from build123d import *

# Parameters (mm, degrees)
ESBO_O1_W                = 63
ESBO_O1_H                = 60
RESSALTO_EXTRUS_O1_DEPTH = 1
RESSALTO_EXTRUS_O2_DEPTH = 1
RESSALTO_EXTRUS_O3_DEPTH = 1


with BuildPart() as part:
    # Esboço1 → Ressalto-extrusão1 (new, symmetric)
    with BuildSketch(Plane.XY):
        Rectangle(ESBO_O1_W, ESBO_O1_H)
    extrude(amount=RESSALTO_EXTRUS_O1_DEPTH, both=True)

    # Esboço2 → Ressalto-extrusão2 (add, symmetric)
    with BuildSketch(Plane(origin=(23.625, 0, -13.63990011), x_dir=(0, -1, 0), z_dir=(-0.8660254037844416, 0, 0.49999999999999495))):
        Polygon((-29.995618948, 75.849181721), (-29.995618948, 15.75), (26.534381052, 15.75), (26.534381052, 20.91864534), (24.774381052, 22.73864534), align=None)
    extrude(amount=RESSALTO_EXTRUS_O2_DEPTH, both=True)

    # Esboço3 → Ressalto-extrusão3 (add, symmetric)
    with BuildSketch(Plane(origin=(-23.625, 0, 13.63990011), x_dir=(0, -1, 0), z_dir=(0.866025403784445, 0, -0.4999999999999889))):
        Polygon((30, 15.75), (-30, 15.75), (-30, 43.326372281), (-36.552202997, 62.375919638), (17.643604412, 43.326372281), align=None)
    extrude(amount=RESSALTO_EXTRUS_O3_DEPTH, both=True)


solid = part.part
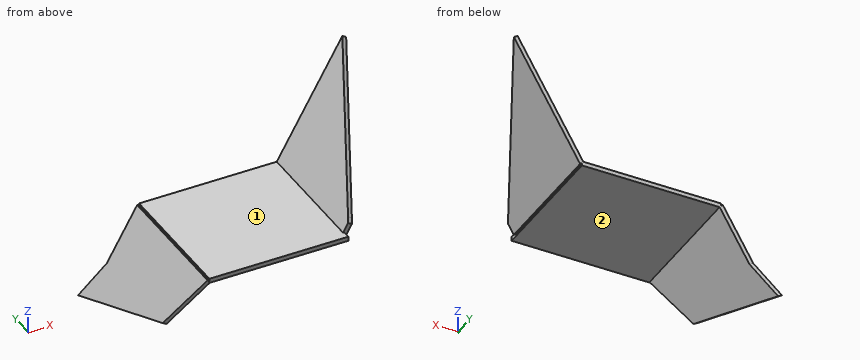
Could you check a few things on this model? Use its own coordinates, in mm. Face numbers are marked on the shaded views. A direction names the side the tool comes from. Coordinates: 2 decimals unless noted, no trailing zeros. Order: outer loops, then holes, each group sorted by start corner. A loop starts at its lowest first (then second) coordinate and runs counter-clockwise, first axis right, second up. Notation, with made-up numbers: (26, 20) - (68, 20) arc R26 ccw to (68, 42) - close; hole circle Ø9 at (-18, 26). An arc over 180 degrees is marked (long way). Answer in a Markdown table with one row per item. Add a question column.
(1) If we section it at B-B, the plane x = 6.5: Please give me the cut outline in (y, z), then the cut area to 3 significant figures.
(2) Will these pins go through, and if not, where does the flat tip stop? pin 1 (18 mm diameter, centred on x = 0.5, y = 4.5, fed in from -Z); pin 2 (9.5 mm diameter, centred on x = 52, z = 26, fed in from +Y); pin 3 (1.6 mm diameter, centred on y = -5.5, z = 0, fed in from +X).
(3) On a 3-axis mill with a long thin cutter (end or side, diameter ignored), from which of +Z, -Z, +X, -X, +Y, -Y can I reach the whole of each face in a straight line? I mean the marked faces 1 and 2. Say none if no direction works.
(4) If we section it at D-D, the plane y = -2: Please give me the cut outline in (x, z).
(5) I need wall thicknesses on L1, parallel to Z at x = -0.5, y = 27; L2, parallel to Y at x = 28.5, z = -0.5; L3, parallel to X at y = -23, z = -7. Which ranges of each line are inside material? Lowest first, please.
(6) If we section it at A-A, the plane y = 12: Please give me the cut outline in (x, z).
(7) If we section it at C-C, the plane z = -8: Please give me the cut outline in (x, y).
Results are:
| question | item | result |
|---|---|---|
| 1 | outline | (-30, -1) - (30, -1) - (30, 1) - (-30, 1) - close |
| 1 | area | 120 mm2 |
| 2 | pin 1 | stops at z = -1 |
| 2 | pin 2 | stops at y = 30 |
| 2 | pin 3 | stops at x = 33.12 |
| 3 | face 1 | +Z, -X, +Y, -Y |
| 3 | face 2 | -Z, +X, +Y, -Y |
| 4 | outline | (-48.9, -28.14) - (-47.17, -29.14) - (-30.92, -1) - (31.5, -1) - (31.5, 0) - (32.37, -0.5) - (46.9, 24.68) - (45.17, 25.68) - (30.92, 1) - (-31.5, 1) - (-31.5, 0) - (-32.37, 0.5) - close |
| 5 | L1 | z = -1 to 1 |
| 5 | L2 | y = -30 to 30 |
| 5 | L3 | x = -36.7 to -34.39 |
| 6 | outline | (-51.36, -32.41) - (-49.63, -33.41) - (-30.92, -1) - (31.5, -1) - (31.5, 0) - (32.37, -0.5) - (53.69, 36.43) - (51.96, 37.43) - (30.92, 1) - (-31.5, 1) - (-31.5, 0) - (-32.37, 0.5) - close |
| 7 | outline | (-37.27, -25.6) - (-34.96, -26.12) - (-34.96, 30) - (-37.27, 30) - close |
